from build123d import *

# Parameters (mm, degrees)
SKETCH1_R                = 60
SKETCH1_R_2              = 4
BOSS_EXTRUDE1_DEPTH      = 3
SKETCH2_W                = 110
SKETCH2_H                = 12
BOSS_EXTRUDE2_DEPTH      = 4
F_5_0_5_DIAMETER_HOLE1_D = 5
SKETCH5_W                = 110
SKETCH5_H                = 100
SKETCH5_R                = 3
BOSS_EXTRUDE3_DEPTH      = 3
BOSS_EXTRUDE4_START      = -3
BOSS_EXTRUDE4_DEPTH      = 3
SKETCH7_W                = 250
SKETCH7_H                = 150
SKETCH7_W_2              = 200
SKETCH7_H_2              = 100
CUT_EXTRUDE1_DEPTH       = 5
CHAMFER1_SIZE            = 20
SKETCH8_R                = 4
CUT_EXTRUDE2_DEPTH       = 15
FILLET1_R                = 10
CUT_EXTRUDE3_START       = -4
SKETCH9_W                = 110
SKETCH9_H                = 12
SKETCH9_R                = 2.5
CUT_EXTRUDE3_DEPTH       = 4


with BuildPart() as part:
    # Sketch1 → Boss-Extrude1 (new body)
    with BuildSketch(Plane.XY):
        Circle(SKETCH1_R)
        with Locations((-37.5, 0)):
            Circle(SKETCH1_R_2, mode=Mode.SUBTRACT)
        with Locations((0, -37.5)):
            Circle(SKETCH1_R_2, mode=Mode.SUBTRACT)
        with Locations((37.5, 0)):
            Circle(SKETCH1_R_2, mode=Mode.SUBTRACT)
        with Locations((0, 37.5)):
            Circle(SKETCH1_R_2, mode=Mode.SUBTRACT)
    extrude(amount=BOSS_EXTRUDE1_DEPTH)

    # Sketch2 → Boss-Extrude2 (add)
    with BuildSketch(Plane.XY.offset(3)):
        with Locations((5, 15)):
            Rectangle(SKETCH2_W, SKETCH2_H)
    extrude(amount=BOSS_EXTRUDE2_DEPTH)

    # Ø5.0 (5) Diameter Hole1 (through all)
    with Locations(Plane.XY.offset(7)):
        with Locations((-15, 15), (15, 15), (-15, -15), (15, -15)):
            Hole(F_5_0_5_DIAMETER_HOLE1_D / 2)

    # Sketch5 → Boss-Extrude3 (add)
    with BuildSketch(Plane.XY.offset(3)):
        with Locations((80, 0)):
            Rectangle(SKETCH5_W, SKETCH5_H)
        with Locations((70, 39.998003983)):
            Circle(SKETCH5_R, mode=Mode.SUBTRACT)
        with Locations((119.99999996, 40)):
            Circle(SKETCH5_R, mode=Mode.SUBTRACT)
        with Locations((119.99999996, -40)):
            Circle(SKETCH5_R, mode=Mode.SUBTRACT)
        with Locations((70, -40.001996017)):
            Circle(SKETCH5_R, mode=Mode.SUBTRACT)
    extrude(amount=-BOSS_EXTRUDE3_DEPTH)

    # Sketch6 → Boss-Extrude4 (add)
    with BuildSketch(Plane.XY.offset(3).offset(BOSS_EXTRUDE4_START)):
        with BuildLine():
            ThreePointArc((-33.166247904, -50), (-60, 0), (-33.166247904, 50))
            Line((-33.166247904, 50), (-65, 50))
            Line((-65, 50), (-65, -50))
            Line((-65, -50), (-33.166247904, -50))
        make_face()
    extrude(amount=BOSS_EXTRUDE4_DEPTH)

    # Sketch7 → Cut-Extrude1 (cut)
    with BuildSketch(Plane.XY.offset(3)):
        with Locations((35, 0)):
            Rectangle(SKETCH7_W, SKETCH7_H)
        with Locations((35, 0)):
            Rectangle(SKETCH7_W_2, SKETCH7_H_2, mode=Mode.SUBTRACT)
    extrude(amount=-CUT_EXTRUDE1_DEPTH, mode=Mode.SUBTRACT)

    # Chamfer1
    chamfer1_edges = [part.edges().sort_by_distance(p)[0] for p in [
        (-65, 50, 1.5),
        (-65, -50, 1.5),
    ]]
    chamfer(chamfer1_edges, length=CHAMFER1_SIZE)

    # Sketch8 → Cut-Extrude2 (cut)
    with BuildSketch(Plane.XY.offset(3)):
        with Locations((37.5, 0)):
            Circle(SKETCH8_R)
    extrude(amount=-CUT_EXTRUDE2_DEPTH, mode=Mode.SUBTRACT)

    # Fillet1
    fillet1_edges = [part.edges().sort_by_distance(p)[0] for p in [
        (-45, 50, 1.5),
        (-65, -30, 1.5),
        (-65, 30, 1.5),
        (-45, -50, 1.5),
        (135, -50, 1.5),
        (135, 50, 1.5),
    ]]
    fillet(fillet1_edges, radius=FILLET1_R)

    # Sketch9 → Cut-Extrude3 (cut)
    with BuildSketch(Plane.XY.offset(7).offset(CUT_EXTRUDE3_START)):
        with Locations((5, 15)):
            Rectangle(SKETCH9_W, SKETCH9_H)
        with Locations((-15, 15)):
            Circle(SKETCH9_R, mode=Mode.SUBTRACT)
        with Locations((15, 15)):
            Circle(SKETCH9_R, mode=Mode.SUBTRACT)
    extrude(amount=CUT_EXTRUDE3_DEPTH, mode=Mode.SUBTRACT)


solid = part.part
CAD build for the part. Positions are in the model's coordinates, mm. Coordinates: 2 decimals unless noted, no trailing zeros. Order: outer loops, then holes, each group sorted by start corner. A loop starts at its lowest first (then second) coordinate and runs counter-clockwise, first axis right, second up. Notation, with made-up numbers: (33, 35) -> (77, 35) arc R28 cw to (77, 59) -> close; hole circle Ø10 at (69.25, -28.75). An arc over 180 degrees is marked (long way). Answer in a Markdown table with one row per item.
1) Band-saw the part on D-D (x = 70). List the corners of the cut face in (y, z).
Check values:
| item | result |
|---|---|
| outline | (-50, 0) -> (-43, 0) -> (-43, 3) -> (-50, 3) -> close; (-37, 0) -> (37, 0) -> (37, 3) -> (-37, 3) -> close; (43, 0) -> (50, 0) -> (50, 3) -> (43, 3) -> close |
2) Band-saw the part on B-B (x = -37.5). List the corners of the cut face in (y, z).
Check values:
| item | result |
|---|---|
| outline | (-50, 0) -> (-4, 0) -> (-4, 3) -> (-50, 3) -> close; (4, 0) -> (50, 0) -> (50, 3) -> (4, 3) -> close |
3) Mould opens along X. For faces 1 (the face through (34, 12, 3)), 2 (the face through (131.99, 47.15, 1.48)), 3 (the face through (-0.521, 41.466, 1.479)), 4 (the face through (-55, -40, 1)) say: pulls with the +X half, pulls with the -X half, needs draft (parallel to the pull), parting line crosses it, or undercut.
Check values:
| item | result |
|---|---|
| face 1 | needs draft |
| face 2 | pulls with the +X half |
| face 3 | undercut |
| face 4 | pulls with the -X half |
4) Band-saw the part on C-C (z = 2.1). Give the number of separate pieces and of enclosed holes in the cut face, and give its area (3 significant figures).
Check values:
| item | result |
|---|---|
| separate pieces | 1 |
| enclosed holes | 12 |
| area | 19,200 mm2 |
5) Band-saw the part on A-A (x = 15). List the corners of the cut face in (y, z), and give its area (3 significant figures).
Check values:
| item | result |
|---|---|
| outline | (-50, 0) -> (-17.5, 0) -> (-17.5, 3) -> (-50, 3) -> close; (-12.5, 0) -> (12.5, 0) -> (12.5, 3) -> (-12.5, 3) -> close; (17.5, 0) -> (50, 0) -> (50, 3) -> (17.5, 3) -> close |
| area | 270 mm2 |
6) Drill centre lines: line 1 (Y direction, x = 120, z = 1.75); line 2 (Y direction, x = 0, z = 1.9); line 3 (X direction, y = 39.5, z = 2.6). Where is each one in solid material? Low to high.
Check values:
| item | result |
|---|---|
| line 1 | -50 to -43, -37 to 37, 43 to 50 |
| line 2 | -50 to -41.5, -33.5 to 33.5, 41.5 to 50 |
| line 3 | -55.5 to -3.46, 3.46 to 67.04, 72.96 to 117.04, 122.96 to 135 |
